```python
from build123d import *

# Parameters (mm, degrees)
SKETCH1_W           = 15
SKETCH1_H           = 90
BOSS_EXTRUDE1_DEPTH = 1.45
SKETCH2_W           = 1.45
SKETCH2_H           = 90
BOSS_EXTRUDE2_DEPTH = 23.55
SKETCH3_R           = 1.5
CUT_EXTRUDE1_DEPTH  = 26
SKETCH5_R           = 1.865
CUT_EXTRUDE2_DEPTH  = 1.45
CUT_EXTRUDE3_REACH  = 17
SKETCH6_R           = 1.5


with BuildPart() as part:
    # Sketch1 → Boss-Extrude1 (new body)
    with BuildSketch(Plane.XY):
        Rectangle(SKETCH1_W, SKETCH1_H)
    extrude(amount=BOSS_EXTRUDE1_DEPTH)

    # Sketch2 → Boss-Extrude2 (add)
    with BuildSketch(Plane.XY.offset(1.45)):
        with Locations((-6.775, 0)):
            Rectangle(SKETCH2_W, SKETCH2_H)
    extrude(amount=BOSS_EXTRUDE2_DEPTH)

    # Sketch3 → Cut-Extrude1 (cut, through all)
    with BuildSketch(Plane(origin=(0, 0, 0), x_dir=(-1, 0, 0), z_dir=(0, 0, -1))):
        with Locations((0, 40)):
            Circle(SKETCH3_R)
        with Locations((0, -40)):
            Circle(SKETCH3_R)
    extrude(amount=-CUT_EXTRUDE1_DEPTH, mode=Mode.SUBTRACT)

    # Sketch5 → Cut-Extrude2 (cut)
    with BuildSketch(Plane.ZY.offset(7.5)):
        with Locations((16.057, -30.462)):
            Circle(SKETCH5_R)
    cut_extrude2 = extrude(amount=-CUT_EXTRUDE2_DEPTH, mode=Mode.SUBTRACT)

    # Mirror1: Cut-Extrude2 across plane
    add(cut_extrude2.mirror(Plane.ZX), mode=Mode.SUBTRACT)

    # Sketch6 → Cut-Extrude3 (cut, up to next)
    with BuildSketch(Plane.ZY.offset(7.5), mode=Mode.PRIVATE) as cut_extrude3_sk1:
        with Locations((10.33, 0)):
            Circle(SKETCH6_R)
    cut_extrude3_tool1 = extrude(cut_extrude3_sk1.sketch, amount=-CUT_EXTRUDE3_REACH, mode=Mode.PRIVATE) & part.part
    add(cut_extrude3_tool1.solids().sort_by_distance((-7.5, 0, 10.33))[0], mode=Mode.SUBTRACT)


solid = part.part
```
Part model, mm, in its own coordinate system. A direction names the side the tool comes from. Round coordinates to 2 decimals unless told otherwise and drop trailing zeros. Write each loop counter-clockwise with the first axis right and the second up, starting at its lowest first coordinate (ties: lowest second). Pieces come first, ordered by that corner, then holes. Notation, with made-up numbers: (-4, -15) -> (11, -15) arc R16 cw to (11, 6) -> close; hole circle Ø9 at (-14, 42.25). An arc over 180 degrees is marked (long way). Return JSON: item names as keys, results as strings. Group by question number.
Q1. Probe L1, parallel to Y at x = 0, z = 0.6; L2, parallel to Y at x = -6.9, z = 10.33; L3, parallel to X at y = 26.5, z = 23.5. List the from-to ranges inside material, lowest first. Write a range as [from, to].
Q2. Saw through at A-A on x = 0. Write the cut outline in (y, z).
Q3. Saw through at D-D on x = 3.5. Write the cut outline in (y, z), plus the area to 4 significant figures.
Q4. Which spindle directions (+Z, -Z, +X, -X, +Y, -Y) get a long thin tool onto all of the face, cutting with end or side? Do faces 4 (the flat face through (-6.05, -1, 13)), 5 (the cylindrical face through (-6.79, -32.28, 15.65)). Say none if no direction does.
Q5. Saw through at C-C on y = -17. Write the cut outline in (x, z), plus the area to 3 significant figures.
Q6. Mould opens along Z. For faces 1 (the flat face through (-7, 45, 9)), 2 (the cylindrical face through (-6.785, -0.575, 11.716)), 3 (the flat face through (-7, 1, 25)) say: pulls with the +Z half, pulls with the -Z half, needs draft (parallel to the pull), parting line crosses it, or undercut.
Q7. Saw through at B-B on y = -40. Write the cut outline in (x, z), plus the area to 3 significant figures.
Q8. Pin check, flat tips, straight feed: pin 1 (8 mm diameter, centred on x = 5.5, y = -7.5, fed in from +Z); pin 2 (2 mm diameter, centred on y = -6, z = 9, fed in from +X); pin 3 (1 mm diameter, centred on x = 4, y = -28.5, fed in from -Z); pin 4 (4 mm diameter, centred on y = -11, z = 18.5, fed in from +X). Stop position of each tip, or through.
Answer:
{
 "1": {"L1": "[-45, -41.5], [-38.5, 38.5], [41.5, 45]", "L2": "[-45, -1.5], [1.5, 45]", "L3": "[-7.5, -6.05]"},
 "2": {"outline": "(-45, 0) -> (-41.5, 0) -> (-41.5, 1.45) -> (-45, 1.45) -> close; (-38.5, 0) -> (38.5, 0) -> (38.5, 1.45) -> (-38.5, 1.45) -> close; (41.5, 0) -> (45, 0) -> (45, 1.45) -> (41.5, 1.45) -> close"},
 "3": {"outline": "(-45, 0) -> (45, 0) -> (45, 1.45) -> (-45, 1.45) -> close", "area": "130.5 mm2"},
 "4": {"face 4": "+Z, +X, +Y, -Y", "face 5": "+X, -X"},
 "5": {"outline": "(-7.5, 0) -> (7.5, 0) -> (7.5, 1.45) -> (-6.05, 1.45) -> (-6.05, 25) -> (-7.5, 25) -> close", "area": "55.9 mm2"},
 "6": {"face 1": "needs draft", "face 2": "undercut", "face 3": "pulls with the +Z half"},
 "7": {"outline": "(-7.5, 0) -> (-1.5, 0) -> (-1.5, 1.45) -> (-6.05, 1.45) -> (-6.05, 25) -> (-7.5, 25) -> close; (1.5, 0) -> (7.5, 0) -> (7.5, 1.45) -> (1.5, 1.45) -> close", "area": "51.5 mm2"},
 "8": {"pin 1": "z = 1.45", "pin 2": "x = -6.05", "pin 3": "z = 0", "pin 4": "x = -6.05"}
}
